```python
from build123d import *

# Parameters (mm, degrees)
BASE_FLANGE1_DEPTH  = 495
SKETCH6_W           = 32.5
SKETCH6_H           = 20
CUT_EXTRUDE1_DEPTH  = 4.5
LPATTERN1_COUNT     = 3
LPATTERN1_PITCH     = 232.5
LPATTERN1_COL_COUNT = 3
LPATTERN1_COL_PITCH = 232.5
SKETCH7_W           = 32.5
SKETCH7_H           = 20
CUT_EXTRUDE2_DEPTH  = 4.5
LPATTERN2_COUNT     = 3
LPATTERN2_PITCH     = 232.5
LPATTERN2_COL_COUNT = 3
LPATTERN2_COL_PITCH = 232.5
SKETCH8_R           = 3
CUT_EXTRUDE3_DEPTH  = 5
LPATTERN3_COUNT     = 3
LPATTERN3_PITCH     = 232.5
LPATTERN3_COL_COUNT = 3
LPATTERN3_COL_PITCH = 232.5
SKETCH9_R           = 3.125
CUT_EXTRUDE4_DEPTH  = 10
LPATTERN4_COUNT     = 3
LPATTERN4_PITCH     = 232.5
LPATTERN4_COL_COUNT = 3
LPATTERN4_COL_PITCH = 232.5


# Sheet-metal steps are written as plain solids
with BuildPart() as part:
    # Sketch1 → Base-Flange1 (new, symmetric)
    with BuildSketch(Plane.XY):
        with BuildLine():
            Line((0, 114), (0, 126.1))
            ThreePointArc((0, 126.1), (-0.556497116, 127.443502884), (-1.9, 128))
            Line((-1.9, 128), (-26.1, 128))
            ThreePointArc((-26.1, 128), (-27.443502884, 127.443502884), (-28, 126.1))
            Line((-28, 126.1), (-28, 19.9))
            ThreePointArc((-28, 19.9), (-27.443502884, 18.556497116), (-26.1, 18))
            Line((-26.1, 18), (-3.9, 18))
            ThreePointArc((-3.9, 18), (-1.142283553, 16.857716447), (0, 14.1))
            Line((0, 14.1), (0, 3.9))
            ThreePointArc((0, 3.9), (-1.142283553, 1.142283553), (-3.9, 0))
            Line((-3.9, 0), (-14, 0))
            Line((-14, 0), (-14, 2))
            Line((-14, 2), (-3.9, 2))
            ThreePointArc((-3.9, 2), (-2.556497116, 2.556497116), (-2, 3.9))
            Line((-2, 3.9), (-2, 14.1))
            ThreePointArc((-2, 14.1), (-2.556497116, 15.443502884), (-3.9, 16))
            Line((-3.9, 16), (-26.1, 16))
            ThreePointArc((-26.1, 16), (-28.857716447, 17.142283553), (-30, 19.9))
            Line((-30, 19.9), (-30, 126.1))
            ThreePointArc((-30, 126.1), (-28.857716447, 128.857716447), (-26.1, 130))
            Line((-26.1, 130), (-1.9, 130))
            ThreePointArc((-1.9, 130), (0.857716447, 128.857716447), (2, 126.1))
            Line((2, 126.1), (2, 114))
            Line((2, 114), (0, 114))
        make_face()
    extrude(amount=BASE_FLANGE1_DEPTH, both=True)

    # Sketch6 → Cut-Extrude1 (cut)
    with BuildSketch(Plane(origin=(0, 130, 0), x_dir=(1, 0, 0), z_dir=(0, 1, 0))):
        with Locations((-14, 0)):
            Rectangle(SKETCH6_W, SKETCH6_H)
    cut_extrude1 = extrude(amount=-CUT_EXTRUDE1_DEPTH, mode=Mode.SUBTRACT)

    # LPattern1: Cut-Extrude1 ×3
    with Locations(*[(0, 0, i * LPATTERN1_PITCH) for i in range(1, LPATTERN1_COUNT)]):
        add(cut_extrude1, mode=Mode.SUBTRACT)

    # LPattern1 col: Cut-Extrude1 ×3
    with Locations(*[(0, 0, -i * LPATTERN1_COL_PITCH) for i in range(1, LPATTERN1_COL_COUNT)]):
        add(cut_extrude1, mode=Mode.SUBTRACT)

    # Sketch7 → Cut-Extrude2 (cut, symmetric)
    with BuildSketch(Plane(origin=(0, 18, 0), x_dir=(1, 0, 0), z_dir=(0, 1, 0))):
        with Locations((-14, 0)):
            Rectangle(SKETCH7_W, SKETCH7_H)
    cut_extrude2 = extrude(amount=CUT_EXTRUDE2_DEPTH, both=True, mode=Mode.SUBTRACT)

    # LPattern2: Cut-Extrude2 ×3
    with Locations(*[(0, 0, -i * LPATTERN2_PITCH) for i in range(1, LPATTERN2_COUNT)]):
        add(cut_extrude2, mode=Mode.SUBTRACT)

    # LPattern2 col: Cut-Extrude2 ×3
    with Locations(*[(0, 0, i * LPATTERN2_COL_PITCH) for i in range(1, LPATTERN2_COL_COUNT)]):
        add(cut_extrude2, mode=Mode.SUBTRACT)

    # Sketch8 → Cut-Extrude3 (cut)
    with BuildSketch(Plane(origin=(0, 2, 0), x_dir=(1, 0, 0), z_dir=(0, 1, 0))):
        with Locations(Location((-8.95, 0, 0), (0, 0, 180))):
            Circle(SKETCH8_R)
    cut_extrude3 = extrude(amount=-CUT_EXTRUDE3_DEPTH, mode=Mode.SUBTRACT)

    # LPattern3: Cut-Extrude3 ×3
    with Locations(*[(0, 0, -i * LPATTERN3_PITCH) for i in range(1, LPATTERN3_COUNT)]):
        add(cut_extrude3, mode=Mode.SUBTRACT)

    # LPattern3 col: Cut-Extrude3 ×3
    with Locations(*[(0, 0, i * LPATTERN3_COL_PITCH) for i in range(1, LPATTERN3_COL_COUNT)]):
        add(cut_extrude3, mode=Mode.SUBTRACT)

    # Sketch9 → Cut-Extrude4 (cut)
    with BuildSketch(Plane.ZY.offset(30)):
        with Locations(Location((0, 104, 0), (0, 0, 270))):
            Circle(SKETCH9_R)
        with Locations(Location((0, 44, 0), (0, 0, 270))):
            Circle(SKETCH9_R)
    cut_extrude4 = extrude(amount=-CUT_EXTRUDE4_DEPTH, mode=Mode.SUBTRACT)

    # LPattern4: Cut-Extrude4 ×3
    with Locations(*[(0, 0, -i * LPATTERN4_PITCH) for i in range(1, LPATTERN4_COUNT)]):
        add(cut_extrude4, mode=Mode.SUBTRACT)

    # LPattern4 col: Cut-Extrude4 ×3
    with Locations(*[(0, 0, i * LPATTERN4_COL_PITCH) for i in range(1, LPATTERN4_COL_COUNT)]):
        add(cut_extrude4, mode=Mode.SUBTRACT)


solid = part.part
```
Here's how the part is built. I have some questions about the finished solid (model axes, mm). A direction names the side the tool comes from. Round coordinates to 2 decimals unless told otherwise and drop trailing zeros. Write each loop counter-clockwise with the first axis right and the second up, starting at its lowest first coordinate (ties: lowest second). Pieces come first, ordered by that corner, then holes.
Q1. If we mould it in two halves opening along X, with no side actions, what happens to faces 5 (the flat face through (-30, 72, 7)), 6 (the flat face through (-14, 128, -115)), 7 (the flat face through (-15, 18, -115))? For each: +X half, -X half, draft (parallel to the pull), parting line (faces both ways), or undercut.
Q2. If we section it at A-A on z = -32.5: Write out the boundary of the cut face in (x, y).
Q3. Which directions (+Z, -Z, +X, -X, +Y, -Y) give clear straight access to the entire face, cutting with the end or side of a thin tool? Please do faces 1 (the flat face through (-15, 16, -115)), 2 (the flat face through (-14, 128, 118)), 3 (the flat face through (-14, 130, 485)), 4 (the flat face through (-15, 18, 118)).
Q4. Will these pins go through, and if not, where does the flat tip stop? P1, Ø2.5, axis at x = -8.5, y = 20, coming from the +Z side; P2, Ø1.6, axis at x = -29, z = -463, coming from the -Y side; P3, Ø2, axis at x = -1.5, z = 82.5, coming from the -Y side; P4, Ø1.6, axis at x = -1, z = 470, coming from the +Y side.
Q5. Please list where these lines run through material, in increasing order: probe 1 along Y at (x, z) = (-4.5, 64.5); probe 2 along Z at (x, y) = (-29.45, 104) (3 decimals); probe 3 along Y at (x, z) = (-15, 113.5).
Q6. If we section it at B-B on y = 57.5: Write out the boundary of the cut face in (x, z).
Answer below:
1. face 5: -X half
1. face 6: undercut
1. face 7: draft
2. outline: (-30, 19.9) arc R3.9 ccw to (-26.1, 16) - (-3.9, 16) arc R1.9 cw to (-2, 14.1) - (-2, 3.9) arc R1.9 cw to (-3.9, 2) - (-14, 2) - (-14, 0) - (-3.9, 0) arc R3.9 ccw to (0, 3.9) - (0, 14.1) arc R3.9 ccw to (-3.9, 18) - (-26.1, 18) arc R1.9 cw to (-28, 19.9) - (-28, 126.1) arc R1.9 cw to (-26.1, 128) - (-1.9, 128) arc R1.9 cw to (0, 126.1) - (0, 114) - (2, 114) - (2, 126.1) arc R3.9 ccw to (-1.9, 130) - (-26.1, 130) arc R3.9 ccw to (-30, 126.1) - close
3. face 1: +Z, -Z, -X
3. face 2: +Z, -Z
3. face 3: +Z, -Z, +X, -X, +Y
3. face 4: +Z, -Z, +X
4. P1: passes through
4. P2: stops at y = 22.5
4. P3: stops at y = 0.26
4. P4: stops at y = 13.5
5. probe 1: y = 0 to 2, 16 to 18, 128 to 130
5. probe 2: z = -495 to -468.125, -461.875 to -235.625, -229.375 to -3.125, 3.125 to 229.375, 235.625 to 461.875, 468.125 to 495
5. probe 3: y = 16 to 18, 128 to 130
6. outline: (-30, -495) - (-28, -495) - (-28, 495) - (-30, 495) - close
